Source: three-view drawing plus pictorial views. Frame: mm from the lowest corner of the part. Give positions to 0.01 mm unless a question says otherwise; leave off trailing zeros. Loops run counter-clockwise (first coordinate to the right, second up) from the corner with the lowest first, then second, coordinate; pieces in that order, holes last. Notation, with made-up numbers: (7, 59) - (63, 59) arc R33 cw to (63, 97) - close; hole circle Ø6 at (33, -4). An arc over 180 degrees is marked (long way). Answer as a JSON object with one key per item and string values. Group by question number.
(1) Section query A-A (y = 5). Return loops of the section in (x, z).
(2) Section query D-D (x = 15). Return loops of the section in (y, z), plus the area to 3 significant figures.
(3) Pin query (flat end, axial travel): P1, Ø9.5, axis at x = 17.5, y = 16, coming from the +Z side; P2, Ø6, axis at x = 19, z = 44, coming from the -Y side; P3, Ø5, axis at x = 24, y = 25.5, coming from the +Z side; P4, Ø8, axis at y = 18, z = 57.5, coming from the +X side. Return the tip coordinate at first contact, or that it passes through.
(4) Material intervals for L1, parallel to Y at x = 25, z = 2.9; L2, parallel to X at y = 15.25, z = 206.5; L3, parallel to Z at x = 22.25, y = 25.25, sorted ascending.
(5) Section query C-C (z = 134.5). Return loops of the section in (x, y).
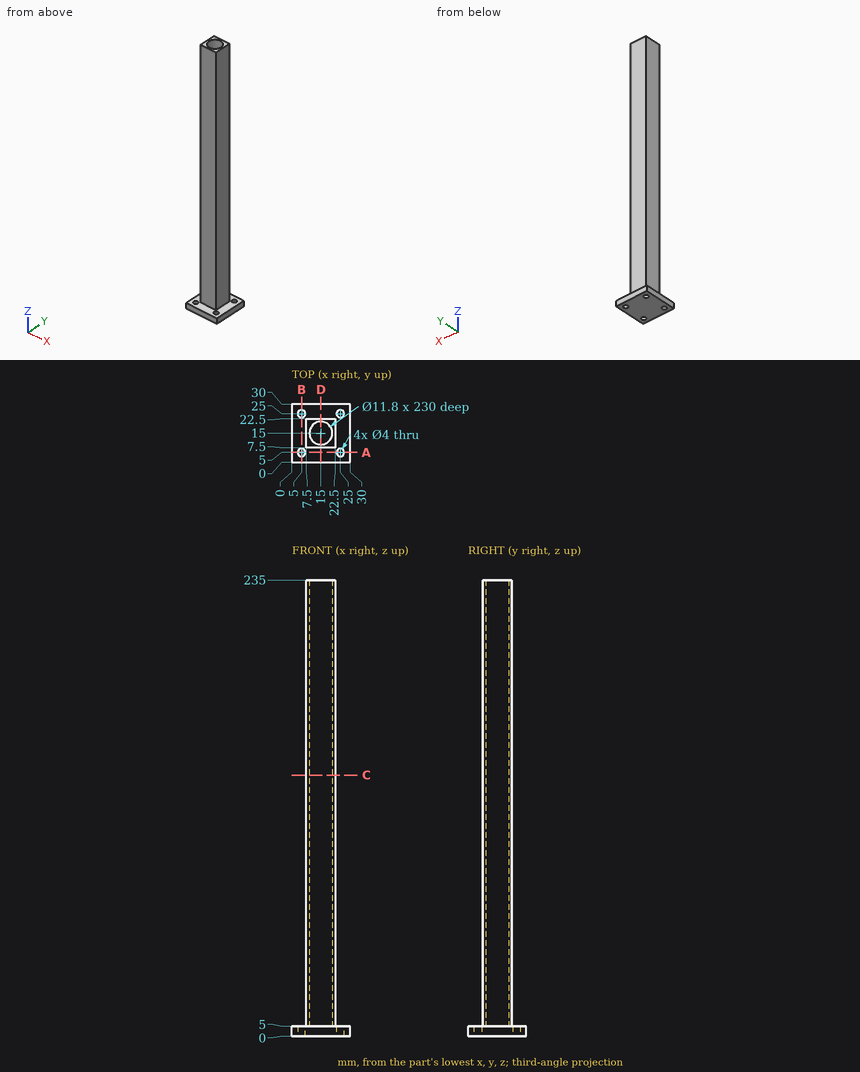
Recorded:
{
 "1": {"outline": "(0, 0) - (3, 0) - (3, 5) - (0, 5) - close; (7, 0) - (23, 0) - (23, 5) - (7, 5) - close; (27, 0) - (30, 0) - (30, 5) - (27, 5) - close"},
 "2": {"outline": "(0, 0) - (30, 0) - (30, 5) - (22.5, 5) - (22.5, 235) - (20.9, 235) - (20.9, 5) - (9.1, 5) - (9.1, 235) - (7.5, 235) - (7.5, 5) - (0, 5) - close", "area": "886 mm^2"},
 "3": {"P1": "stops at z = 235", "P2": "stops at y = 7.5", "P3": "stops at z = 5", "P4": "stops at x = 22.5"},
 "4": {"L1": "y = 0 to 3, 7 to 23, 27 to 30", "L2": "x = 7.5 to 9.11, 20.89 to 22.5", "L3": "z = 0 to 5"},
 "5": {"outline": "(7.5, 7.5) - (22.5, 7.5) - (22.5, 22.5) - (7.5, 22.5) - close; hole circle Ø11.8 at (15, 15)"}
}
